Source: CAD feature listing. Evaluate the final solid. Frame: model axes, mm. Face numbers are marked on the shaded views. Round coordinates to 2 decimals unless told otherwise and drop trailing zeros. Loops run counter-clockwise (first coordinate to the right, second up) from the corner with the lowest first, then second, coordinate; pieces in that order, holes last. Notation, with made-up numbers: M -23,-37 L 23,-37 A19 ccw 23,-17 Z; hole C 62,3 d11. An arc over 180 degrees is marked long. Answer as a JSON object with one key per item and string values.
from build123d import *

# Parameters (mm, degrees)
SKETCH_1_R      = 1.65
EXTRUDE_1_DEPTH = 3


with BuildPart() as part:
    # 草图1 → 凸台-拉伸1 (new body)
    with BuildSketch(Plane.XY):
        with BuildLine():
            ThreePointArc((-16, 2.4), (-18.4, 0), (-16, -2.4))
            Line((-16, -2.4), (0, -3.7))
            Line((0, -3.7), (16, -2.4))
            ThreePointArc((16, -2.4), (18.4, 0), (16, 2.4))
            Line((16, 2.4), (0, 3.7))
            Line((0, 3.7), (-16, 2.4))
        make_face()
        with Locations((-16, 0)):
            Circle(SKETCH_1_R, mode=Mode.SUBTRACT)
        Circle(SKETCH_1_R, mode=Mode.SUBTRACT)
        with Locations((16, 0)):
            Circle(SKETCH_1_R, mode=Mode.SUBTRACT)
    extrude(amount=EXTRUDE_1_DEPTH)


solid = part.part
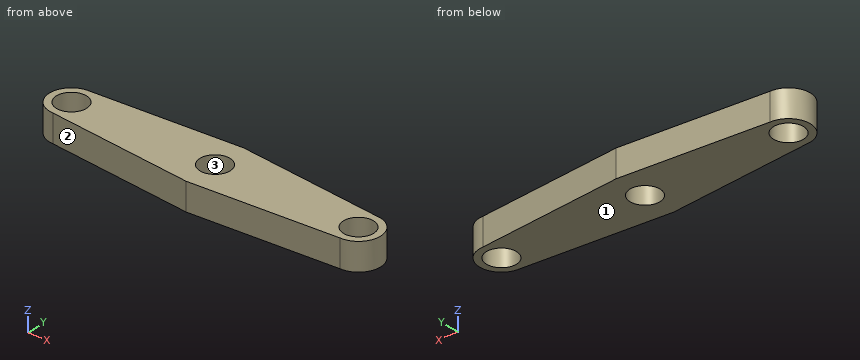
Item 1: Section A-A on y = 0. Return the cut outline in (x, z).
Answer sheet:
{"outline": "M -18.4,0 L -17.65,0 L -17.65,3 L -18.4,3 Z; M -14.35,0 L -1.65,0 L -1.65,3 L -14.35,3 Z; M 1.65,0 L 14.35,0 L 14.35,3 L 1.65,3 Z; M 17.65,0 L 18.4,0 L 18.4,3 L 17.65,3 Z"}
Item 2: Pull-direction query (X, two-part tool) for the marked faces 1, 2 and 3; classes: pulls with the +X half, pulls with the -X half, needs draft (parallel to the pull), parting line crosses it, or undercut.
Answer sheet:
{"face 1": "needs draft", "face 2": "pulls with the -X half", "face 3": "undercut"}
Item 3: Section C-C on x = 8. Return the cut outline in (y, z), then the cut area to 3 significant figures.
Answer sheet:
{"outline": "M -3.05,0 L 3.05,0 L 3.05,3 L -3.05,3 Z", "area": "18.3 mm²"}
Item 4: Line query: probe 1 along Y at (x, z) = (-16, 1.4); probe 2 along X at (y, z) = (-0.75, 0.2); probe 3 along X at (y, z) = (0.5, 2.6). Output: solid intervals per line, ascending. Write a range as from..to.
Answer sheet:
{"probe 1": "y = -2.4..-1.65, 1.65..2.4", "probe 2": "x = -18.28..-17.47, -14.53..-1.47, 1.47..14.53, 17.47..18.28", "probe 3": "x = -18.35..-17.57, -14.43..-1.57, 1.57..14.43, 17.57..18.35"}
Item 5: Section B-B on z = 0.8. Return the cut outline in (x, y), then the cut area to 3 significant figures.
Answer sheet:
{"outline": "M -16,-2.4 L 0,-3.7 L 16,-2.4 A2.4 ccw 16,2.4 L 0,3.7 L -16,2.4 A2.4 ccw Z; hole C -16,0 d3.3; hole C 0,0 d3.3; hole C 16,0 d3.3", "area": "188 mm²"}
Item 6: Section D-D on y = -3. Return the cut outline in (x, z), then the cut area to 3 significant figures.
Answer sheet:
{"outline": "M -8.62,0 L 8.62,0 L 8.62,3 L -8.62,3 Z", "area": "51.7 mm²"}
Item 7: Contact query for flat-ended pins moving along their axis: pin 1 Ø3 at (x, y) = (-10.5, 2) entering from -Z; pin 2 Ø1 at (y, z) = (1.5, 1.5) entering from +X; pin 3 Ø1.5 at (x, z) = (5, 2.5) entering from -Y. Output: stop coordinate, or through.
Answer sheet:
{"pin 1": "stops at z = 0", "pin 2": "stops at x = 18.18", "pin 3": "stops at y = -3.35"}
